Study the drawing (mm; zero at the part's minimum x, y, z) and answer. A direction names the side the tool comes from. Give positions to 0.01 mm unless a question says otherwise; leave off trailing zeros. Order: outer loops, then holes, each group sorted by start corner. A loop starts at its lowest first (then second) coordinate and runs counter-clockwise, first axis right, second up. Notation, with made-up numbers: (-16, 12) -> (38, 12) arc R25 cw to (38, 35) -> close; hole circle Ø9 at (-25.5, 37.5). An arc over 180 degrees is marked (long way). Answer as CSV lines item,"result". Start each with the question number.
1. A cutting plane is placed at B-B (z = 17.9). Give the vertices of the cut face in (x, y).
2. Find the intervals of material crossed by L1, parallel to Z at x = 36.3, y = 0.5; L2, parallel to Z at x = 6.5, y = 0.4; L3, parallel to X at y = 3.25, z = 12.75, in increasing order.
3. For the marked faces 4, 5, 6, 7 and 8, determine the directions among +Z, -Z, +X, -X, +Y, -Y from which every point of the face is accessible in a straight line to the end or side of a thin tool.
4. A cutting plane is placed at D-D (y = 7.25). Give the vertices of the cut face in (x, z), then the cut area to 3 significant figures.
5. A cutting plane is placed at C-C (x = 30.5). Give the vertices of the cut face in (y, z), then the cut area to 3 significant figures.
6. Flat-ended cylindrical pins translate along their axes: pin 1 (3.5 mm diameter, centred on x = 16, z = 7, fed in from +Y); pin 2 (3 mm diameter, centred on x = 11, y = 6, fed in from -Z); pin 3 (2.5 mm diameter, centred on x = 36.3, z = 17.9, fed in from +Y); pin 4 (2 mm diameter, centred on y = 7, z = 17.5, fed in from -X). Find the tip coordinate at first contact, or state that the pin passes through.
7. A cutting plane is placed at A-A (y = 3.75). Give the vertices of the cut face in (x, z).
8. For a pull along X with two mould halves and no side action, classify the marked faces 1, 2 and 3 as released by +X, released by -X, zero draft, split by the parting line, or undercut.
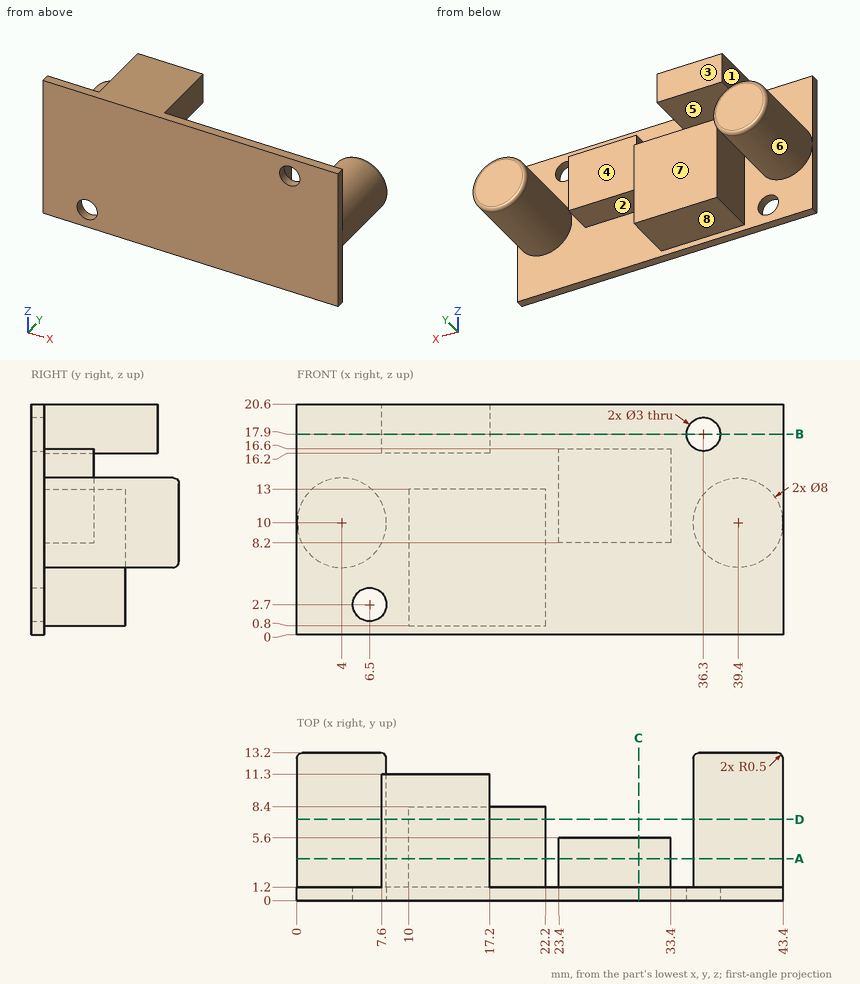
Answer sheet:
1,outline,"(0, 0) -> (34.8, 0) -> (34.8, 1.2) -> (17.2, 1.2) -> (17.2, 11.3) -> (7.6, 11.3) -> (7.6, 1.2) -> (0, 1.2) -> close; (37.8, 0) -> (43.4, 0) -> (43.4, 1.2) -> (37.8, 1.2) -> close"
2,L1,"z = 0 to 16.4, 19.4 to 20.6"
2,L2,"z = 0 to 1.2, 4.2 to 20.6"
2,L3,"x = 1.1 to 6.9, 10 to 22.2, 23.4 to 33.4, 36.5 to 42.3"
3,face 4,"+Z, -Z, +Y"
3,face 5,"-X, +Y"
3,face 6,"+Y"
3,face 7,"-Z, +Y"
3,face 8,"-Z, +X, -X, +Y"
4,outline,"circle Ø8 at (4, 10); (7.6, 16.2) -> (17.2, 16.2) -> (17.2, 20.6) -> (7.6, 20.6) -> close; (10, 0.8) -> (22.2, 0.8) -> (22.2, 13) -> (10, 13) -> close; circle Ø8 at (39.4, 10)"
4,area,"292 mm^2"
5,outline,"(0, 0) -> (1.2, 0) -> (1.2, 8.2) -> (5.6, 8.2) -> (5.6, 16.6) -> (1.2, 16.6) -> (1.2, 20.6) -> (0, 20.6) -> close"
5,area,"61.7 mm^2"
6,pin 1,"stops at y = 8.4"
6,pin 2,"stops at z = 0.8"
6,pin 3,"passes through"
6,pin 4,"stops at x = 7.6"
7,outline,"circle Ø8 at (4, 10); (7.6, 16.2) -> (17.2, 16.2) -> (17.2, 20.6) -> (7.6, 20.6) -> close; (10, 0.8) -> (22.2, 0.8) -> (22.2, 13) -> (10, 13) -> close; (23.4, 8.2) -> (33.4, 8.2) -> (33.4, 16.6) -> (23.4, 16.6) -> close; circle Ø8 at (39.4, 10)"
8,face 1,"released by -X"
8,face 2,"undercut"
8,face 3,"zero draft"
